from build123d import *

# Parameters (mm, degrees)
SKETCH_1_W          = 16
SKETCH_1_H          = 18
EXTRUDE_1_DEPTH     = 1
SKETCH_2_W          = 15.6
SKETCH_2_H          = 15.6
EXTRUDE_2_DEPTH     = 1
SKETCH_3_R          = 7.8
EXTRUDE_3_DEPTH     = 15
EXTRUDE_4_DEPTH     = 3
SKETCH_5_R          = 4
EXTRUDE_5_DEPTH     = 4
SKETCH_7_R          = 0.5
CUT_EXTRUDE_1_DEPTH = 15
SKETCH_8_W          = 1.5
SKETCH_8_H          = 5.6
EXTRUDE_6_DEPTH     = 2
SKETCH_9_R          = 2
SKETCH_10_R         = 1.7
SKETCH_11_R         = 0.5
CUT_EXTRUDE_2_DEPTH = 11
SKETCH_12_W         = 16
SKETCH_12_H         = 1
EXTRUDE_7_DEPTH     = 19
SKETCH_13_R         = 4.1
EXTRUDE_8_DEPTH     = 2
SKETCH_14_W         = 1.5
SKETCH_14_H         = 5.8
CUT_EXTRUDE_3_DEPTH = 1
FILLET_1_R          = 0.4
FILLET_2_R          = 0.4


with BuildPart() as part:
    # 草图1 → 凸台-拉伸1 (new body)
    with BuildSketch(Plane(origin=(0, 0, 0), x_dir=(1, 0, 0), z_dir=(0, 1, 0))):
        Rectangle(SKETCH_1_W, SKETCH_1_H)
    extrude(amount=EXTRUDE_1_DEPTH)

    # 草图2 → 凸台-拉伸2 (add)
    with BuildSketch(Plane(origin=(0, 1, 0), x_dir=(1, 0, 0), z_dir=(0, 1, 0))):
        Rectangle(SKETCH_2_W, SKETCH_2_H)
    extrude(amount=EXTRUDE_2_DEPTH)

    # 草图3 → 凸台-拉伸3 (add)
    with BuildSketch(Plane(origin=(0, 2, 0), x_dir=(1, 0, 0), z_dir=(0, 1, 0))):
        with Locations(Location((0, 0, 0), (0, 0, 270))):
            Circle(SKETCH_3_R)
    extrude(amount=EXTRUDE_3_DEPTH)

    # 草图4 → 凸台-拉伸4 (add)
    with BuildSketch(Plane(origin=(0, 17, 0), x_dir=(1, 0, 0), z_dir=(0, 1, 0))):
        Polygon((-4.8, 7.8), (4.8, 7.8), (4.8, 5.8), (7.8, 2.8), (7.8, -2.8), (4.8, -5.8), (4.8, -7.8), (-4.8, -7.8), (-4.8, -5.8), (-7.8, -2.8), (-7.8, 2.8), (-4.8, 5.8), align=None)
    extrude(amount=EXTRUDE_4_DEPTH)

    # 草图5 → 凸台-拉伸5 (add)
    with BuildSketch(Plane(origin=(0, 20, 0), x_dir=(1, 0, 0), z_dir=(0, 1, 0))):
        with Locations(Location((0, 0, 0), (0, 0, 90))):
            Circle(SKETCH_5_R)
    extrude(amount=EXTRUDE_5_DEPTH)

    # 草图6 → 旋转1 (revolve)
    with BuildSketch(Plane.XY, mode=Mode.PRIVATE) as revolve_1_sk:
        Polygon((0, 24), (4, 24), (2, 25), (1.7, 35), (0, 35), align=None)
    revolve(revolve_1_sk.sketch.rotate(Axis((0, 35, 0), (0, -1, 0)), 270), axis=Axis((0, 35, 0), (0, -1, 0)))

    # 草图7 → 切除-拉伸1 (cut)
    with BuildSketch(Plane(origin=(0, 35, 0), x_dir=(1, 0, 0), z_dir=(0, 1, 0))):
        with Locations(Location((0, 0, 0), (0, 0, 180))):
            Circle(SKETCH_7_R)
    extrude(amount=-CUT_EXTRUDE_1_DEPTH, mode=Mode.SUBTRACT)

    # 草图8 → 凸台-拉伸6 (add)
    with BuildSketch(Plane(origin=(0, 20, 0), x_dir=(1, 0, 0), z_dir=(0, 1, 0))):
        with Locations((7.05, 0)):
            Rectangle(SKETCH_8_W, SKETCH_8_H)
    extrude(amount=EXTRUDE_6_DEPTH)

    # 草图9 → 放样1 section 0
    with BuildSketch(Plane(origin=(7.8, 0, 0), x_dir=(0, 0, -1), z_dir=(1, 0, 0))):
        with Locations((0, 19.5)):
            Circle(SKETCH_9_R)
    # 草图10 → 放样1 section 1
    with BuildSketch(Plane(origin=(17.8, 0, 0), x_dir=(0, 0, -1), z_dir=(1, 0, 0))):
        with Locations((0, 19.5)):
            Circle(SKETCH_10_R)
    loft()

    # 草图11 → 切除-拉伸2 (cut)
    with BuildSketch(Plane(origin=(17.8, 0, 0), x_dir=(0, 0, -1), z_dir=(1, 0, 0))):
        with Locations((0, 19.5)):
            Circle(SKETCH_11_R)
    extrude(amount=-CUT_EXTRUDE_2_DEPTH, mode=Mode.SUBTRACT)

    # 草图12 → 凸台-拉伸7 (add)
    with BuildSketch(Plane(origin=(0, 1, 0), x_dir=(1, 0, 0), z_dir=(0, 1, 0))):
        with Locations((0, 8.5)):
            Rectangle(SKETCH_12_W, SKETCH_12_H)
        with Locations((0, -8.5)):
            Rectangle(SKETCH_12_W, SKETCH_12_H)
    extrude(amount=EXTRUDE_7_DEPTH)

    # 草图13 → 凸台-拉伸8 (add)
    with BuildSketch(Plane(origin=(0, 20, 0), x_dir=(1, 0, 0), z_dir=(0, 1, 0))):
        Polygon((8, 2.9), (6.2, 2.9), (6.2, -2.9), (8, -2.9), (8, -9), (-8, -9), (-8, 9), (8, 9), align=None)
        with Locations(Location((0, 0, 0), (0, 0, 270))):
            Circle(SKETCH_13_R, mode=Mode.SUBTRACT)
    extrude(amount=EXTRUDE_8_DEPTH)

    # 草图14 → 切除-拉伸3 (cut)
    with BuildSketch(Plane(origin=(0, 22, 0), x_dir=(1, 0, 0), z_dir=(0, 1, 0))):
        with Locations((-7.25, 0)):
            Rectangle(SKETCH_14_W, SKETCH_14_H)
    extrude(amount=-CUT_EXTRUDE_3_DEPTH, mode=Mode.SUBTRACT)

    # 圆角1
    fillet_1_edges = [part.edges().sort_by_distance(p)[0] for p in [
        (7.8, 19.5, 2),
        (0, 25, 2),
    ]]
    fillet(fillet_1_edges, radius=FILLET_1_R)

    # 圆角2
    fillet_2_edges = [part.edges().sort_by_distance(p)[0] for p in [
        (0, 22, 9),
        (0, 22, -9),
    ]]
    fillet(fillet_2_edges, radius=FILLET_2_R)


solid = part.part
Could you check a few things on this model? Use its own coordinates, in mm. A direction names the side the tool comes from. Give positions to 0.01 mm unless a question says otherwise; leave off trailing zeros. Order: outer loops, then holes, each group sorted by start corner. A loop starts at its lowest first (then second) coordinate and runs counter-clockwise, first axis right, second up.
Item 1: If we mould it in two halves opening along Y, with no side actions, what happens to faces 1 (the face through (-7, 21, 0)), 2 (the face through (-6.3, 18.5, -4.3))? For each: pulls with the +Y half, pulls with the -Y half, needs draft (parallel to the pull), parting line crosses it, or undercut.
Item 2: I'm going to push flat-ended pins straight in: pin 1 (8 mm diameter, centred on x = 14, z = -5.5, fed in from -Y); pin 2 (1.5 mm diameter, centred on y = 15.5, z = -3.5, fed in from -X); pin 3 (2 mm diameter, centred on x = 5.5, z = -4.5, fed in from +Y). Where does each tip first touch, or does it pass through?
Item 3: If we section it at C-C, the plane z = 5: Write out the boundary of the cut face in (x, y).
Item 4: For faces 3 (the face through (0, 18, 7.8)), 4 (the face through (7, 20, 4)), 5 (the face through (-7.6, 17, 2.4)), which set-ups out of +Z, -Z, +X, -X, +Y, -Y let a thin tool reach every point of the face, with its end or its side?
Item 5: If we section it at B-B, the plane x = 5.75: Write out the boundary of the cut face in (y, z), plus the area to 3 significant figures.
Item 6: I need wall thicknesses on line 1 (Y direction, x = 6.5, z = -6.25); line 2 (X direction, y = 18.5, z = 2.5); line 3 (Z direction, x = 0, y = 24.25). Which ranges of each line are inside material? Lowest first, please.
Item 7: If we section it at D-D, the plane y = 19.5: Count the separate pieces of the cut face and the enclosed holes in it, plus the area to 3 significant figures.
Item 8: If we section it at A-A, the plane y = 29: Write out the boundary of the cut face in (x, z), plus the area to 3 significant figures.
Values:
1. face 1: pulls with the +Y half
1. face 2: undercut
2. pin 1: stops at y = 18.48
2. pin 2: stops at x = -7.3
2. pin 3: stops at y = 22
3. outline: (-8, 0) - (8, 0) - (8, 1) - (7.8, 1) - (7.8, 2) - (5.99, 2) - (5.99, 17) - (5.6, 17) - (5.6, 20) - (8, 20) - (8, 22) - (-8, 22) - (-8, 20) - (-5.6, 20) - (-5.6, 17) - (-5.99, 17) - (-5.99, 2) - (-7.8, 2) - (-7.8, 1) - (-8, 1) - close
4. face 3: +X, -X
4. face 4: none
4. face 5: -X
5. outline: (0, -9) - (21.6, -9) arc R0.4 ccw to (22, -8.6) - (22, 8.6) arc R0.4 ccw to (21.6, 9) - (0, 9) - close; hole (1, -8) - (20, -8) - (20, -4.85) - (17, -4.85) - (17, -5.27) - (2, -5.27) - (2, -7.8) - (1, -7.8) - close; hole (1, 7.8) - (2, 7.8) - (2, 5.27) - (17, 5.27) - (17, 4.85) - (20, 4.85) - (20, 8) - (1, 8) - close
5. area: 295 mm2
6. line 1: y = 0 to 2, 20 to 22
6. line 2: x = -7.8 to 7.8
6. line 3: z = -3.5 to -0.5, 0.5 to 3.5
7. separate pieces: 3
7. enclosed holes: 0
7. area: 259 mm2
8. outline: circle Ø3.76 at (0, 0); hole circle Ø1 at (0, 0)
8. area: 10.3 mm2
